```python
from build123d import *

# Parameters (mm, degrees)
SKETCH1_R           = 3.683
BOSS_EXTRUDE1_DEPTH = 12.7
SKETCH3_R           = 4
BOSS_EXTRUDE3_DEPTH = 12.7
SKETCH2_R           = 3.683
SKETCH2_R_2         = 4
BOSS_EXTRUDE2_DEPTH = 6.35
SKETCH4_R           = 3.2385
CUT_EXTRUDE1_DEPTH  = 139.431456414


with BuildPart() as part:
    # Sketch1 → Boss-Extrude1 (new body)
    with BuildSketch(Plane.XY):
        with BuildLine():
            Line((93.98, -12.7), (-93.98, -12.7))
            ThreePointArc((-93.98, -12.7), (-96.674076836, -11.584076836), (-97.79, -8.89))
            Line((-97.79, -8.89), (-97.79, 8.89))
            ThreePointArc((-97.79, 8.89), (-96.674076836, 11.584076836), (-93.98, 12.7))
            Line((-93.98, 12.7), (93.98, 12.7))
            ThreePointArc((93.98, 12.7), (96.674076836, 11.584076836), (97.79, 8.89))
            Line((97.79, 8.89), (97.79, -8.89))
            ThreePointArc((97.79, -8.89), (96.674076836, -11.584076836), (93.98, -12.7))
        make_face()
        with Locations((-88.9, 0)):
            Circle(SKETCH1_R, mode=Mode.SUBTRACT)
        with Locations((88.9, 0)):
            Circle(SKETCH1_R, mode=Mode.SUBTRACT)
    extrude(amount=BOSS_EXTRUDE1_DEPTH)

    # Sketch3 → Boss-Extrude3 (add, through all)
    with BuildSketch(Plane.XY.offset(12.7)):
        with BuildLine():
            Line((-6.335384206, -97.155), (6.335384206, -97.155))
            ThreePointArc((6.335384206, -97.155), (9.927486654, -95.667102448), (11.415384206, -92.075))
            Line((11.415384206, -92.075), (11.415384206, 92.075))
            ThreePointArc((11.415384206, 92.075), (9.927486654, 95.667102448), (6.335384206, 97.155))
            Line((6.335384206, 97.155), (-6.335384206, 97.155))
            ThreePointArc((-6.335384206, 97.155), (-9.927486654, 95.667102448), (-11.415384206, 92.075))
            Line((-11.415384206, 92.075), (-11.415384206, -92.075))
            ThreePointArc((-11.415384206, -92.075), (-9.927486654, -95.667102448), (-6.335384206, -97.155))
        make_face()
        with Locations((0, 88.9)):
            Circle(SKETCH3_R, mode=Mode.SUBTRACT)
        with Locations((0, -88.9)):
            Circle(SKETCH3_R, mode=Mode.SUBTRACT)
    extrude(amount=-BOSS_EXTRUDE3_DEPTH)

    # Sketch2 → Boss-Extrude2 (add)
    with BuildSketch(Plane(origin=(0, 0, 0), x_dir=(-1, 0, 0), z_dir=(0, 0, -1))):
        with Locations((-88.9, 0)):
            Circle(SKETCH2_R)
        with Locations((88.9, 0)):
            Circle(SKETCH2_R)
        with Locations(Location((0, 88.9, 0), (0, 0, 180))):
            Circle(SKETCH2_R_2)
        with Locations(Location((0, -88.9, 0), (0, 0, 180))):
            Circle(SKETCH2_R_2)
    extrude(amount=-BOSS_EXTRUDE2_DEPTH)

    # Sketch4 → Cut-Extrude1 (cut, through all)
    with BuildSketch(Plane.XY.offset(12.7)):
        with Locations((-68.58, 0)):
            Circle(SKETCH4_R)
        with Locations((0, 68.58)):
            Circle(SKETCH4_R)
        with Locations((68.58, 0)):
            Circle(SKETCH4_R)
        with Locations((0, -68.58)):
            Circle(SKETCH4_R)
    extrude(amount=-CUT_EXTRUDE1_DEPTH, mode=Mode.SUBTRACT)


solid = part.part
```
The listing builds one solid part. Answer for the finished solid, in the listing's coordinates (mm). A direction names the side the tool comes from. Give positions to 0.01 mm unless a question says otherwise; leave off trailing zeros. Order: outer loops, then holes, each group sorted by start corner. A loop starts at its lowest first (then second) coordinate and runs counter-clockwise, first axis right, second up. Notation, with made-up numbers: (6.25, -1) -> (32.25, -1) arc R18 cw to (32.25, 19) -> close; hole circle Ø2 at (-12.75, -8). An arc over 180 degrees is marked (long way). Answer as a JSON object with one key per item and string values. Group by question number.
Item 1: The part is cut by section D-D on y = 88.9. Write down the section's boundary in (x, z).
Item 2: The part is cut by section B-B on y = 0. Write down the section's boundary in (x, z), and give its area (3 significant figures).
Item 3: Determine the mould class of faces 1 (the flat face through (97.79, 0, 6)), 2 (the cylindrical face through (9.967, 95.627, 6.439)), 3 (the flat face through (0, -97.155, 6)), 4 (the flat face through (0, 89, 6.35)) for opening direction Y: pulls with the +Y half, pulls with the -Y half, needs draft (parallel to the pull), parting line crosses it, or undercut.
Item 4: A tool of negligible diameter and unlimited length cuts with its end or side. For faces 5 (the flat face through (11.415, 52, 6)), 6 (the flat face through (-89, 0, 6.35)), 7 (the flat face through (-53, 12.7, 6)), from which of +Z, -Z, +X, -X, +Y, -Y can it reach the whole face along a straight path? Write none if from no direction.
Item 5: The part is cut by section C-C on x = 68.58. Write down the section's boundary in (y, z).
Item 6: Flat-ended cylindrical pins translate along their axes: pin 1 (5 mm diameter, centred on x = 0, y = 68.58, fed in from -Z); pin 2 (6.5 mm diameter, centred on x = -42.5, z = 4.5, fed in from -Y); pin 3 (3 mm diameter, centred on y = -15, z = 10, fed in from +X); pin 4 (4 mm diameter, centred on y = 69.5, z = 4, fed in from -X). Find the tip coordinate at first contact, or state that the pin passes through.
Item 7: Consider L1, parallel to Y at x = 0, z = 8 (1 decimal); L2, parallel to Y at x = 0, z = 4.5 (1 decimal); L3, parallel to X at y = 88.9, z = 11.5. Determine where each line is inside the solid, lowest interval first. Write a range as from..to.
Item 8: The part is cut by section A-A on z = 8.5. Give the number of separate pieces and of enclosed holes in the cut face, and give its area (3 significant figures).
Result set:
{
 "1": {"outline": "(-11.42, 0) -> (11.42, 0) -> (11.42, 12.7) -> (4, 12.7) -> (4, 6.35) -> (-4, 6.35) -> (-4, 12.7) -> (-11.42, 12.7) -> close"},
 "2": {"outline": "(-97.79, 0) -> (-71.82, 0) -> (-71.82, 12.7) -> (-85.22, 12.7) -> (-85.22, 6.35) -> (-92.58, 6.35) -> (-92.58, 12.7) -> (-97.79, 12.7) -> close; (-65.34, 0) -> (65.34, 0) -> (65.34, 12.7) -> (-65.34, 12.7) -> close; (71.82, 0) -> (97.79, 0) -> (97.79, 12.7) -> (92.58, 12.7) -> (92.58, 6.35) -> (85.22, 6.35) -> (85.22, 12.7) -> (71.82, 12.7) -> close", "area": "2,230 mm²"},
 "3": {"face 1": "needs draft", "face 2": "pulls with the +Y half", "face 3": "pulls with the -Y half", "face 4": "undercut"},
 "4": {"face 5": "+Z, -Z, +X, +Y", "face 6": "+Z", "face 7": "+Z, -Z, -X, +Y"},
 "5": {"outline": "(-12.7, 0) -> (-3.24, 0) -> (-3.24, 12.7) -> (-12.7, 12.7) -> close; (3.24, 0) -> (12.7, 0) -> (12.7, 12.7) -> (3.24, 12.7) -> close"},
 "6": {"pin 1": "through", "pin 2": "y = -12.7", "pin 3": "x = 11.42", "pin 4": "x = -11.42"},
 "7": {"L1": "-97.2..-92.9, -84.9..-71.8, -65.3..65.3, 71.8..84.9, 92.9..97.2", "L2": "-97.2..-71.8, -65.3..65.3, 71.8..97.2", "L3": "-11.42..-4, 4..11.42"},
 "8": {"separate pieces": "1", "enclosed holes": "8", "area": "8,470 mm²"}
}
